For this review, use the dimensioned drawing (mm, ordinates from the lowest corner) and the shaded views. Give positions to 0.01 mm unless a question says otherwise; leave off trailing zeros. Order: outer loops, then holes, each group sorted by start corner. A loop starts at its lowest first (then second) coordinate and runs counter-clockwise, first axis right, second up.
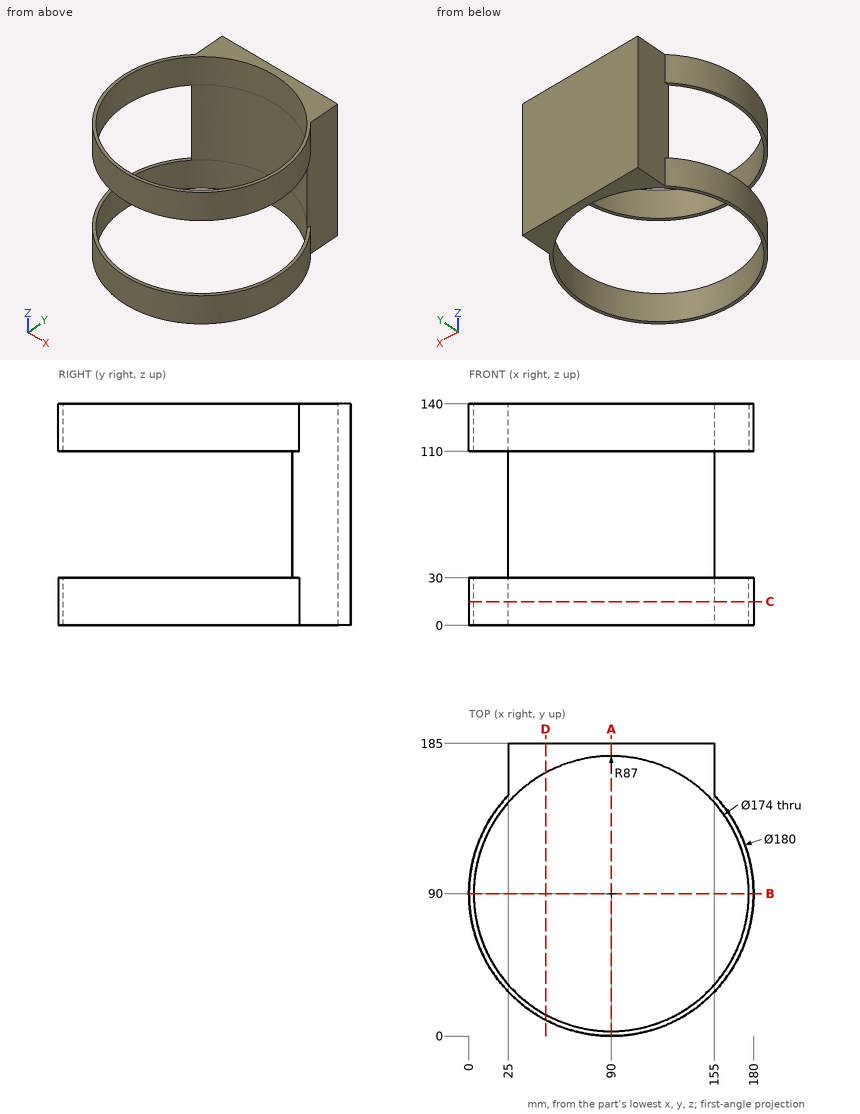
1. Take a section at A-A (x = 90). State the section outline as (y, z) points, then the cut area to 3 significant figures.
Recorded:
outline: (0, 0) - (3, 0) - (3, 30) - (0, 30) - close; (0, 110) - (3, 110) - (3, 140) - (0, 140) - close; (177, 0) - (185, 0) - (185, 140) - (177, 140) - close
area: 1,300 mm2
2. Take a section at C-C (z = 15). State the section outline as (x, y) points, then the cut area to 3 significant figures.
Recorded:
outline: (25, 152.25) arc R90 ccw (long way) to (155, 152.25) - (155, 185) - (25, 185) - close; hole circle Ø174 at (90, 90)
area: 3,440 mm2
3. For pin 1 (1 mm diameter, centred on x = 42.5, z = 87.5, fed in from -Y), flat-tipped, find the tip position at first contact; note if it passes through.
Recorded:
pin 1: stops at y = 162.56
4. For line 1 along X through (y, z) = (90, 13); line 2 along Y through (x, z) = (108, 113); line 3 along Y through (x, z) = (65, 119.5), list the stretches that pass through material, from the lowest coordinate up.
Recorded:
line 1: x = 0 to 3, 177 to 180
line 2: y = 1.82 to 4.88, 175.12 to 185
line 3: y = 3.54 to 6.67, 173.33 to 185
5. Take a section at B-B (y = 90). State the section outline as (x, z) points.
Recorded:
outline: (0, 0) - (3, 0) - (3, 30) - (0, 30) - close; (0, 110) - (3, 110) - (3, 140) - (0, 140) - close; (177, 0) - (180, 0) - (180, 30) - (177, 30) - close; (177, 110) - (180, 110) - (180, 140) - (177, 140) - close
6. Take a section at D-D (x = 48.5). State the section outline as (y, z) points, then the cut area to 3 significant figures.
Recorded:
outline: (10.14, 0) - (13.54, 0) - (13.54, 30) - (10.14, 30) - close; (10.14, 110) - (13.54, 110) - (13.54, 140) - (10.14, 140) - close; (166.46, 0) - (185, 0) - (185, 140) - (166.46, 140) - close
area: 2,800 mm2
